Could you check a few things on this model? Use its own coordinates, in mm. Give positions to 0.01 mm unless a question says otherwise; leave off trailing zeros. Loops run counter-clockwise (first coordinate to the right, second up) from the corner with the lowest first, then second, coordinate; pieces in that order, holes last. Notation, with made-up numbers: (-18, -1.5) -> (-7, -1.5) arc R17 ccw to (-7, 31.5) -> close; hole circle Ø9 at (15.5, -0.75). An arc over 180 degrees is marked (long way). Put each result on its own line as item: value.
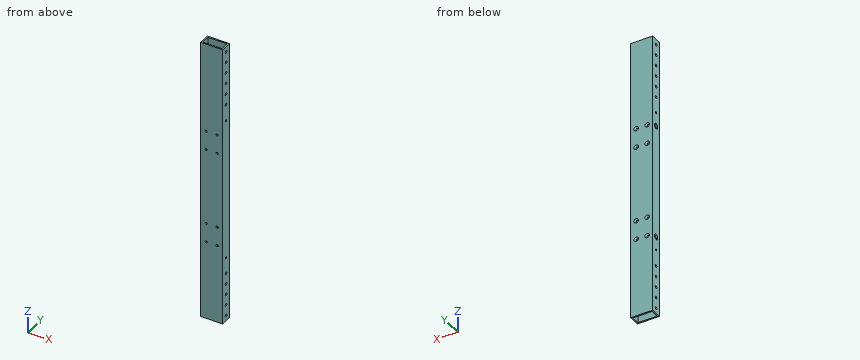
```python
from build123d import *

# Parameters (mm, degrees)
BOSS_EXTRUDE1_DEPTH              = 330.2
BOSS_EXTRUDE1_DEPTH_BACK         = 330.2
SKETCH3_W                        = 50.8
SKETCH3_H                        = 25.4
SKETCH3_W_2                      = 44.45
SKETCH3_H_2                      = 19.05
F_1_4_0_25_DIAMETER_HOLE3_D      = 6.35
F_1_4_0_25_DIAMETER_HOLE4_D      = 6.35
F_1_4_0_25_DIAMETER_HOLE5_D      = 6.35
F_1_4_0_25_DIAMETER_HOLE6_D      = 6.35
F_1_4_0_25_DIAMETER_HOLE7_D      = 6.35
F_1_4_0_25_DIAMETER_HOLE8_D      = 6.35
F_13_64_0_20313_DIAMETER_HOLE1_D = 5.159502
F_1_2_0_5_DIAMETER_HOLE1_D       = 12.7
F_1_2_0_5_DIAMETER_HOLE1_DEPTH   = 6.35
F_1_2_0_5_DIAMETER_HOLE1_TIP     = 3.815464931
F_10_CLEARANCE_HOLE1_AT_2_COUNT  = 2
F_10_CLEARANCE_HOLE1_AT_2_PITCH  = 25.4
F_10_CLEARANCE_HOLE1_AT_3_COUNT  = 2
F_10_CLEARANCE_HOLE1_AT_3_PITCH  = 51.195336702
F_10_CLEARANCE_HOLE1_AT_4_COUNT  = 2
F_10_CLEARANCE_HOLE1_AT_4_PITCH  = 44.45
F_10_CLEARANCE_HOLE1_AT_5_COUNT  = 2
F_10_CLEARANCE_HOLE1_AT_5_PITCH  = 223.596969524
F_10_CLEARANCE_HOLE1_AT_6_COUNT  = 2
F_10_CLEARANCE_HOLE1_AT_6_PITCH  = 222.1496
F_10_CLEARANCE_HOLE1_AT_7_COUNT  = 2
F_10_CLEARANCE_HOLE1_AT_7_PITCH  = 266.5996
F_10_CLEARANCE_HOLE1_AT_8_COUNT  = 2
F_10_CLEARANCE_HOLE1_AT_8_PITCH  = 267.806845917


with BuildPart() as part:
    # Sketch3 → Boss-Extrude1 (new, two sides: drawn at the far end of the back side and taken through both)
    with BuildSketch(Plane.XY.offset(-BOSS_EXTRUDE1_DEPTH_BACK)):
        Rectangle(SKETCH3_W, SKETCH3_H)
        Rectangle(SKETCH3_W_2, SKETCH3_H_2, mode=Mode.SUBTRACT)
    extrude(amount=BOSS_EXTRUDE1_DEPTH + BOSS_EXTRUDE1_DEPTH_BACK)

    # 1/4 (0.25) Diameter Hole3 (through all)
    with Locations(Plane.ZY.offset(25.4)):
        with Locations((-317.5, 0)):
            Hole(F_1_4_0_25_DIAMETER_HOLE3_D / 2)

    # 1/4 (0.25) Diameter Hole4 (through all)
    with Locations(Plane.ZY.offset(25.4)):
        with Locations((292.1, 0), (317.5, 0)):
            Hole(F_1_4_0_25_DIAMETER_HOLE4_D / 2)

    # 1/4 (0.25) Diameter Hole5 (through all)
    with Locations(Plane(origin=(25.4, 0, 0), x_dir=(0, 0, -1), z_dir=(1, 0, 0))):
        with Locations((292.1, 0), (266.7, 0)):
            Hole(F_1_4_0_25_DIAMETER_HOLE5_D / 2)

    # 1/4 (0.25) Diameter Hole6 (through all)
    with Locations(Plane(origin=(25.4, 0, 0), x_dir=(0, 0, -1), z_dir=(1, 0, 0))):
        with Locations((215.9, 0), (241.3, 0)):
            Hole(F_1_4_0_25_DIAMETER_HOLE6_D / 2)

    # 1/4 (0.25) Diameter Hole7 (through all)
    with Locations(Plane(origin=(25.4, 0, 0), x_dir=(0, 0, -1), z_dir=(1, 0, 0))):
        with Locations((-190.5, 0), (-215.9, 0)):
            Hole(F_1_4_0_25_DIAMETER_HOLE7_D / 2)

    # 1/4 (0.25) Diameter Hole8 (through all)
    with Locations(Plane(origin=(25.4, 0, 0), x_dir=(0, 0, -1), z_dir=(1, 0, 0))):
        with Locations((-266.7, 0), (-241.3, 0)):
            Hole(F_1_4_0_25_DIAMETER_HOLE8_D / 2)

    # 13/64 (0.20313) Diameter Hole1 (through all)
    with Locations(Plane(origin=(25.4, 0, 0), x_dir=(0, 0, -1), z_dir=(1, 0, 0))):
        with Locations((-152.4, 0), (177.8, 0)):
            Hole(F_13_64_0_20313_DIAMETER_HOLE1_D / 2)

    # 1/2 (0.5) Diameter Hole1
    with Locations(Plane.ZY.offset(25.4)):
        with Locations((-146.050000508, 4.9e-08), (120.65, 1.7e-08)):
            Hole(F_1_2_0_5_DIAMETER_HOLE1_D / 2, depth=F_1_2_0_5_DIAMETER_HOLE1_DEPTH)
            with Locations((0, 0, -(F_1_2_0_5_DIAMETER_HOLE1_DEPTH + F_1_2_0_5_DIAMETER_HOLE1_TIP / 2))):  # 118° drill point
                Cone(0, F_1_2_0_5_DIAMETER_HOLE1_D / 2, F_1_2_0_5_DIAMETER_HOLE1_TIP, mode=Mode.SUBTRACT)

    # Sketch40 → #10 Clearance Hole1 (revolve, cut)
    with BuildSketch(Plane(origin=(-12.7, -12.7, -145.9998), x_dir=(0, 0, -1), z_dir=(1, 0, 0))):
        Polygon((0, 0), (0, 25.4), (5.2197, 25.4), (2.4892, 22.258919064), (2.4892, 0), align=None)
    f_10_clearance_hole1 = revolve(axis=Axis((-12.7, -19.05, -145.9998), (0, 1, 0)), mode=Mode.SUBTRACT)

    # #10 Clearance Hole1 at 2: #10 Clearance Hole1 ×2
    with Locations(*[(i * F_10_CLEARANCE_HOLE1_AT_2_PITCH, 0, 0) for i in range(1, F_10_CLEARANCE_HOLE1_AT_2_COUNT)]):
        add(f_10_clearance_hole1, mode=Mode.SUBTRACT)

    # #10 Clearance Hole1 at 3: #10 Clearance Hole1 ×2
    with Locations(*[Vector(0.4961389383568339, 0, 0.8682431421244592) * (i * F_10_CLEARANCE_HOLE1_AT_3_PITCH) for i in range(1, F_10_CLEARANCE_HOLE1_AT_3_COUNT)]):
        add(f_10_clearance_hole1, mode=Mode.SUBTRACT)

    # #10 Clearance Hole1 at 4: #10 Clearance Hole1 ×2
    with Locations(*[(0, 0, i * F_10_CLEARANCE_HOLE1_AT_4_PITCH) for i in range(1, F_10_CLEARANCE_HOLE1_AT_4_COUNT)]):
        add(f_10_clearance_hole1, mode=Mode.SUBTRACT)

    # #10 Clearance Hole1 at 5: #10 Clearance Hole1 ×2
    with Locations(*[Vector(0.11359724621542587, 0, 0.9935268821991039) * (i * F_10_CLEARANCE_HOLE1_AT_5_PITCH) for i in range(1, F_10_CLEARANCE_HOLE1_AT_5_COUNT)]):
        add(f_10_clearance_hole1, mode=Mode.SUBTRACT)

    # #10 Clearance Hole1 at 6: #10 Clearance Hole1 ×2
    with Locations(*[(0, 0, i * F_10_CLEARANCE_HOLE1_AT_6_PITCH) for i in range(1, F_10_CLEARANCE_HOLE1_AT_6_COUNT)]):
        add(f_10_clearance_hole1, mode=Mode.SUBTRACT)

    # #10 Clearance Hole1 at 7: #10 Clearance Hole1 ×2
    with Locations(*[(0, 0, i * F_10_CLEARANCE_HOLE1_AT_7_PITCH) for i in range(1, F_10_CLEARANCE_HOLE1_AT_7_COUNT)]):
        add(f_10_clearance_hole1, mode=Mode.SUBTRACT)

    # #10 Clearance Hole1 at 8: #10 Clearance Hole1 ×2
    with Locations(*[Vector(0.09484447611114116, 0, 0.9954921021038807) * (i * F_10_CLEARANCE_HOLE1_AT_8_PITCH) for i in range(1, F_10_CLEARANCE_HOLE1_AT_8_COUNT)]):
        add(f_10_clearance_hole1, mode=Mode.SUBTRACT)


solid = part.part
```
1. I need wall thicknesses on line 1 (Z direction, x = -12.7, y = -10.95); line 2 (Y direction, x = 17.5, z = 81.5) (3 decimals); line 3 (Y direction, x = -23.6, z = 152.4). Which ranges of each line are inside material? Lowest first, please.
Recorded:
line 1: z = -330.2 to -148.49, -143.51 to -104.04, -99.06 to 73.66, 78.64 to 118.11, 123.09 to 330.2
line 2: y = -12.7 to -9.525, 9.525 to 12.7
line 3: y = -12.7 to -2.58, 2.58 to 12.7
2. If we section it at A-A (z = -230): List the corners of the cut face in (x, y) for me (3 decimals).
Recorded:
outline: (-25.4, -12.7) -> (25.4, -12.7) -> (25.4, 12.7) -> (-25.4, 12.7) -> close; hole (-22.225, -9.525) -> (22.225, -9.525) -> (22.225, 9.525) -> (-22.225, 9.525) -> close
3. I'm going to push flat-ended pins straight in: pin 1 (3 mm diameter, centred on x = 12.7, z = -146, fed in from +Y); pin 2 (8 mm diameter, centred on x = 12.7, z = 76.15, fed in from +Y); pin 3 (1 mm diameter, centred on x = 9.5, z = -146.5, fed in from +Y). Where does each tip first touch, or does it pass through?
Recorded:
pin 1: passes through
pin 2: stops at y = 11.3
pin 3: stops at y = 11
